Autodesk Inventor part; units mm, degrees
ref_plane "YZ Plane" through (0, 0, 0) normal (1, 0, 0) x (0, 1, 0)
ref_plane "XZ Plane" through (0, 0, 0) normal (0, 1, 0) x (-1, 0, 0)
ref_plane "XY Plane" through (0, 0, 0) normal (0, 0, 1) x (1, 0, 0)
sketch "Sketch1" plane through (0, 0, 0) normal (0, 0, 1) x (1, 0, 0)
  circle A0 centre (0, 0) radius 2.2479
  circle A1 centre (38.1, 0) radius 2.2479
  circle A2 centre (31.7852, 24.6214) radius 2.0955
  arc A3 (-3.8886, 5.0201) -> (-0.1468, -6.3483) centre (0, 0) ccw
  arc A4 (34.9548, 30.1237) -> (27.8966, 29.6414) centre (31.7852, 24.6214) ccw
  line L0 (-3.8886, 5.0201) -> (27.8966, 29.6414)
  line L1 (38.1, 0) -> (63.5, 0) construction
  circle A5 centre (22.225, -19.05) radius 2.0955
  arc A6 (17.6269, -20.2907) -> (25.681, -22.3268) centre (22.225, -19.05) ccw
  arc A7 (17.6269, -20.2907) -> (-0.1468, -6.3483) centre (-0.5827, -25.2041) ccw
  line L2 (37.8478, -9.4949) -> (25.681, -22.3268)
  circle A8 centre (60.325, 11.1125) radius 2.2479
  arc A9 (62.3683, 7.8968) -> (62.2268, 14.4139) centre (60.325, 11.1125) ccw
  line L3 (62.2268, 14.4139) -> (34.9548, 30.1237)
  line L4 (62.3683, 7.8968) -> (47.4674, -1.5713)
  arc A10 (47.4674, -1.5713) -> (37.8478, -9.4949) centre (74.7114, -44.448) ccw
  point P0 (42.1679, -4.9387)
  dimension "d0" = 4.4958
  dimension "d5" = 12.7
  dimension "d6" = 12.7
  dimension "d14" = 9.525
  dimension "d16" = 7.62
  dimension "d17" = 50.8
extrude "Extrusion1" add sketch "Sketch1" along normal blind 1.5875
properties part number "odom_pod" material "Acetal Resin, White"
Here's how the part is built. I have some questions about the finished solid (model axes, mm). Round coordinates to 2 decimals unless told otherwise and drop trailing zeros. Order: outer loops, then holes, each group sorted by start corner. A loop starts at its lowest first (then second) coordinate and runs counter-clockwise, first axis right, second up. Notation, with made-up numbers: M 14.25,22.5 L 23.25,22.5 A25 ccw 23.25,59.5 Z; hole C 0,-31 d4. An arc over 180 degrees is marked long. One line per question, with ' | ' between items.
1) I want a section at C-C, the plane z = 1.2. State how many separate pieces and enclosed holes the cut face has, then the cut area to 3 significant figures.
Working result:
separate pieces: 1 | enclosed holes: 5 | area: 1,910 mm²
2) I want a section at B-B, the plane y = 0. Write out the boundary of the cut face in (x, z), then the cut area to 3 significant figures.
Working result:
outline: M -6.35,0 L -2.25,0 L -2.25,1.59 L -6.35,1.59 Z; M 2.25,0 L 35.85,0 L 35.85,1.59 L 2.25,1.59 Z; M 40.35,0 L 49.94,0 L 49.94,1.59 L 40.35,1.59 Z | area: 75.1 mm²
3) I want a section at D-D, the plane y = -19.05. Write out the boundary of the cut face in (x, z).
Working result:
outline: M 17.25,0 L 20.13,0 L 20.13,1.59 L 17.25,1.59 Z; M 24.32,0 L 28.79,0 L 28.79,1.59 L 24.32,1.59 Z
4) I need wall thicknesses on line 1 along X through (y, z) = (-2, 0.9); line 2 along X through (y, z) = (-17.5, 0.6); line 3 along X through (y, z) = (-20, 0.25). Which ranges of each line are inside material? Lowest first, please.
Working result:
line 1: -6.03 to -1.03, 1.03 to 37.07, 39.13 to 46.8 | line 2: 16.63 to 20.81, 23.64 to 30.26 | line 3: 17.55 to 20.36, 24.09 to 27.89
5) I want a section at A-A, the plane x = 33. Write out the boundary of the cut face in (y, z), then the cut area to 3 significant figures.
Working result:
outline: M -14.61,0 L 22.91,0 L 22.91,1.59 L -14.61,1.59 Z; M 26.33,0 L 30.85,0 L 30.85,1.59 L 26.33,1.59 Z | area: 66.7 mm²
6) If we mould it in two halves opening along Y, with no side actions, what happens to faces 1 (the face through (11.782, 17.158, 0.783)), 2 (the face through (-5.997, -2.089, 0.783)), 3 (the face through (20.562, -17.775, 0.783)), 4 (the face through (28, 4, 0))? For each: +Y half, -Y half, draft (parallel to the pull), parting line (faces both ways), or undercut.
Working result:
face 1: +Y half | face 2: parting line | face 3: undercut | face 4: draft
7) For pin 1 Ø6.5 at (x, y) = (31.79, 24.62) entering from +Z, with a flat end and sliding along its axis, tell me the tip position at first contact or that it passes through.
Working result:
pin 1: z = 1.59
